Could you check a few things on this model? Use its own coordinates, in mm. Face numbers are marked on the shaded views. A direction names the side the tool comes from. Coordinates: 2 decimals unless noted, no trailing zeros. Loops run counter-clockwise (first coordinate to the right, second up) from the corner with the lowest first, then second, coordinate; pieces in that order, holes last. Notation, with made-up numbers: (-16, -10.5) - (19, -10.5) arc R8 cw to (19, -2.5) - close; hole circle Ø3 at (5.5, -37). An arc over 180 degrees is marked (long way). One line per item, written item: value. Start each with the question number.
(1) On a 3-axis mill with a long thin cutter (end or side, diameter ignored), from which of +Z, -Z, +X, -X, +Y, -Y can I reach the whole of each face in a straight line? I mean the marked faces 1, 2, 3 and 4. Say none if no direction works.
(2) If we section it at C-C on x = 13: Write out the boundary of the cut face in (y, z), then the cut area to 3 significant figures.
(3) If we section it at B-B on z = 4: Write out the boundary of the cut face in (x, y), then the cut area to 3 significant figures.
(4) If we mould it in two halves opening along Y, with no side actions, what happens to the marked faces 5, 6 and 7? For each: pulls with the +Y half, pulls with the -Y half, needs draft (parallel to the pull), parting line crosses it, or undercut.
(5) If we section it at A-A on x = 0: Write out the boundary of the cut face in (y, z).
(6) If we section it at D-D on y = -45: Write out the boundary of the cut face in (x, z).
(7) If I drill on line 1 along Y through (x, z) = (0, 0.75); line 2 along Y through (x, z) = (16, 9.5); line 3 along Y through (x, z) = (56.5, 8.5), over which ranges is the centre line in solid material (lowest first)? Write a range as from..to.
(8) I'm going to push flat-ended pins straight in: P1, Ø6, axis at y = 22.5, z = 2, coming from the -X side; P2, Ø9, axis at x = 15.72, y = -70.77, coming from the -Z side; P3, Ø4, axis at x = 40.5, z = 6.5, coming from the -Y side; P4, Ø1.5, axis at x = 42, z = 8.5, coming from the -Y side. Where does each tip first touch, or does it pass through?
```python
from build123d import *

# Parameters (mm, degrees)
SKETCH1_R           = 5
BOSS_EXTRUDE1_DEPTH = 10
CUT_EXTRUDE1_DEPTH  = 10
CUT_EXTRUDE2_DEPTH  = 10
CUT_EXTRUDE3_DEPTH  = 10
BOSS_EXTRUDE2_DEPTH = 15
SKETCH6_R           = 5
CUT_EXTRUDE4_DEPTH  = 10


with BuildPart() as part:
    # Sketch1 → Boss-Extrude1 (new body)
    with BuildSketch(Plane.XY):
        Polygon((-48.4220718, 40), (-17.320508076, -100), (29.627689013, -100), (29.627689013, -5.894941242), (72.353358785, 40), (54.770735732, 40), align=None)
        Circle(SKETCH1_R, mode=Mode.SUBTRACT)
    extrude(amount=BOSS_EXTRUDE1_DEPTH)

    # Sketch2 → Cut-Extrude1 (cut)
    with BuildSketch(Plane(origin=(0, 0, 0), x_dir=(-1, 0, 0), z_dir=(0, 0, -1))):
        Polygon((44.084731449, 20.475976883), (34.322719891, 22.644647058), (29.98537954, 3.120623941), (39.747391098, 0.951953766), align=None)
        Polygon((25.648039189, -16.403399176), (35.410050747, -18.572069352), (31.072710396, -38.096092469), (21.310698838, -35.927422293), align=None)
        Polygon((16.973358487, -55.45144541), (26.735370045, -57.620115586), (22.398029694, -77.144138703), (12.636018136, -74.975468528), align=None)
    extrude(amount=-CUT_EXTRUDE1_DEPTH, mode=Mode.SUBTRACT)

    # Sketch3 → Cut-Extrude2 (cut)
    with BuildSketch(Plane(origin=(11.20335331, -10.42970665, 12.614201102), x_dir=(-0.825201513, -0.359925431, 0.435311551), z_dir=(-0.564838439, 0.525833566, -0.635969023))):
        Polygon((-74.103118428, 30.827331886), (-22.327074543, -4.543132752), (-17.973959037, 1.829050982), (-4.444119228, 21.634320346), (-66.914441787, 64.310511288), (-84.797397101, 38.133058189), align=None)
    extrude(amount=-CUT_EXTRUDE2_DEPTH, mode=Mode.SUBTRACT)

    # Sketch4 → Cut-Extrude3 (cut)
    with BuildSketch(Plane(origin=(21.723952902, 0, 13.103449585), x_dir=(-0.516496434, 0, 0.85628934), z_dir=(-0.85628934, 0, -0.516496434))):
        Polygon((-3.624300151, -0.279668559), (-15.302595712, -5.894941242), (-15.302595712, -100), (-3.624300151, -100), align=None)
    extrude(amount=-CUT_EXTRUDE3_DEPTH, mode=Mode.SUBTRACT)

    # Sketch5 → Boss-Extrude2 (add)
    with BuildSketch(Plane(origin=(0, 40, 0), x_dir=(1, 0, 0), z_dir=(0, 1, 0))):
        Polygon((72.353358785, 0), (76.20595319, 0), (76.20595319, -10), (61.094050297, -10), (39.843773505, -10), (39.843773505, 0), (61.094050297, 0), align=None)
    extrude(amount=-BOSS_EXTRUDE2_DEPTH)

    # Sketch6 → Cut-Extrude4 (cut)
    with BuildSketch(Plane(origin=(0, 0, 0), x_dir=(-1, 0, 0), z_dir=(0, 0, -1))):
        with Locations((-15.722858772, -70.7745838)):
            Circle(SKETCH6_R)
    extrude(amount=-CUT_EXTRUDE4_DEPTH, mode=Mode.SUBTRACT)


solid = part.part
```
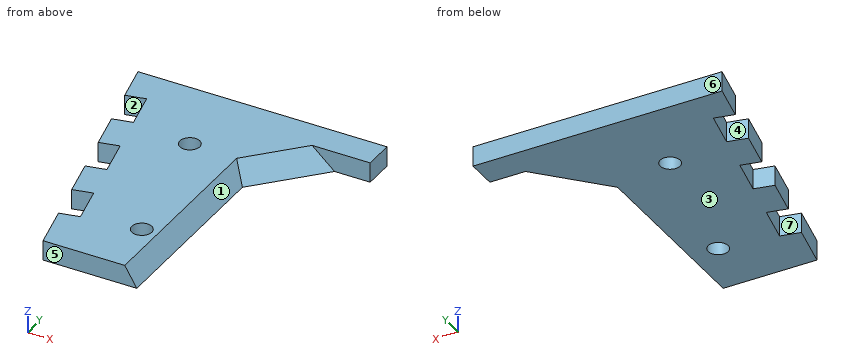
Values:
1. face 1: +Z, +X, -Y
1. face 2: +Z, -Z
1. face 3: -Z, +X, -X, +Y, -Y
1. face 4: +Z, -Z, -X
2. outline: (-100, 0) - (-74.97, 0) - (-74.97, 10) - (-100, 10) - close; (-66.58, 0) - (40, 0) - (40, 10) - (-66.58, 10) - close
2. area: 1,320 mm2
3. outline: (-48.42, 40) - (-44.08, 20.48) - (-34.32, 22.64) - (-29.99, 3.12) - (-39.75, 0.95) - (-35.41, -18.57) - (-25.65, -16.4) - (-21.31, -35.93) - (-31.07, -38.1) - (-26.74, -57.62) - (-16.97, -55.45) - (-12.64, -74.98) - (-22.4, -77.14) - (-17.32, -100) - (27.21, -100) - (27.21, -3.65) - (53.89, 25) - (76.21, 25) - (76.21, 40) - close; hole circle Ø10 at (0, 0); hole circle Ø10 at (15.72, -70.77)
3. area: 8,770 mm2
4. face 5: pulls with the -Y half
4. face 6: pulls with the +Y half
4. face 7: undercut
5. outline: (-100, 0) - (-5, 0) - (-5, 10) - (-100, 10) - close; (5, 0) - (40, 0) - (40, 10) - (5, 10) - close
6. outline: (-29.54, 0) - (29.63, 0) - (23.6, 10) - (-29.54, 10) - close
7. line 1: y = -100..-5, 5..40
7. line 2: y = -100..-75.77, -65.78..40
7. line 3: y = 25..40
8. P1: stops at x = -45.2
8. P2: passes through
8. P3: stops at y = 10.41
8. P4: stops at y = 16.46
